Job drawing, mm, ordinate dimensions from the low corner. One solid piece. A direction names the side the tool comes from. Round coordinates to 2 decimals unless told otherwise and drop trailing zeros. Loops run counter-clockwise (first coordinate to the right, second up) from the corner with the lowest first, then second, coordinate; pieces in that order, holes last.
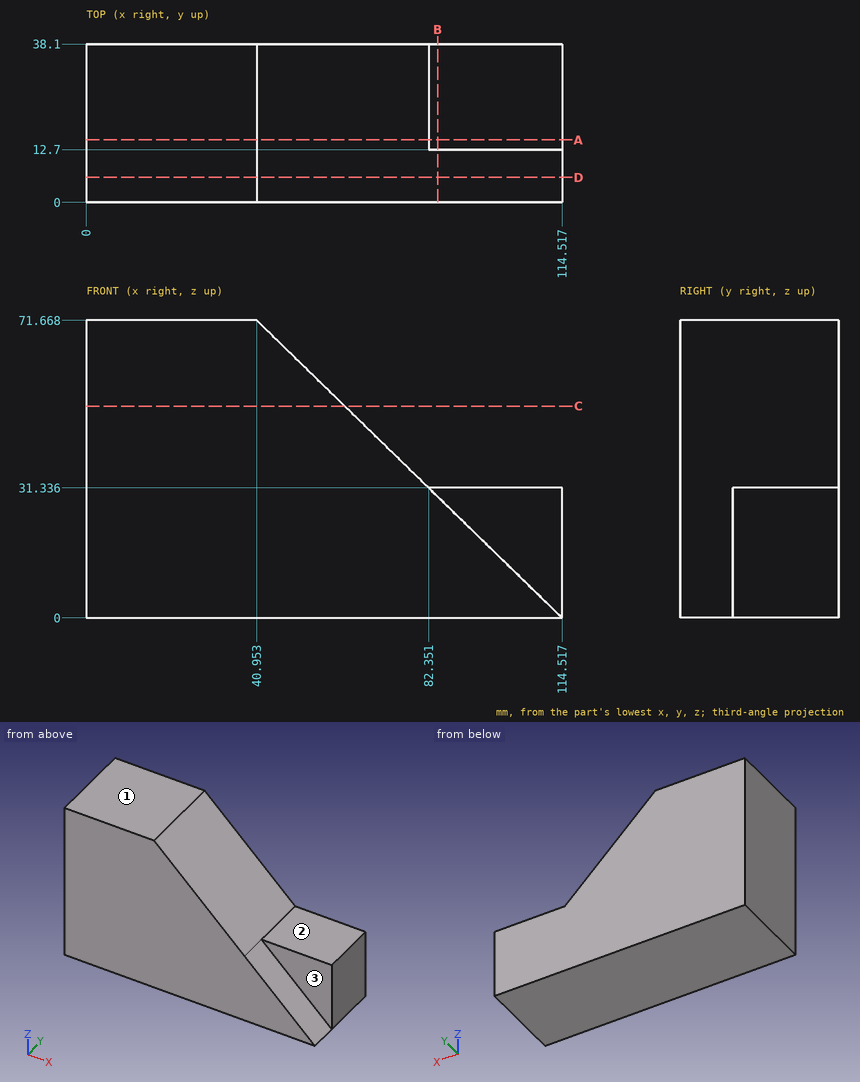
Item 1: Cut at B-B, the plane x = 84.5. Give the cut face in (y, z).
Answers follow:
outline: (0, 0) - (38.1, 0) - (38.1, 31.34) - (12.7, 31.34) - (12.7, 29.24) - (0, 29.24) - close
Item 2: Cut at C-C, the plane z = 51. Give the cut face in (x, y), plus the area to 3 significant figures.
Answers follow:
outline: (0, 0) - (62.17, 0) - (62.17, 38.1) - (0, 38.1) - close
area: 2,370 mm2
Item 3: 3-axis set-ups, long thin cutter, end or side, ignore diameter. For the marked faces 1, 2 and 3: which of +Z, -Z, +X, -X, +Y, -Y reach the whole face in a straight line?
Answers follow:
face 1: +Z, +X, -X, +Y, -Y
face 2: +Z, +X, +Y, -Y
face 3: +Z, +X, -Y
Item 4: Cut at A-A, the plane y = 15. Give the cut face in (x, z), plus the area to 4 significant figures.
Answers follow:
outline: (0, 0) - (114.52, 0) - (114.52, 31.34) - (82.35, 31.34) - (40.95, 71.67) - (0, 71.67) - close
area: 6,075 mm2
Item 5: Probe line 1 (Z direction, x = 104, y = 21); line 2 (Z direction, x = 46, y = 11); line 3 (X direction, y = 24, z = 66). List the from-to ranges inside material, lowest first.
Answers follow:
line 1: z = 0 to 31.34
line 2: z = 0 to 66.75
line 3: x = 0 to 46.77
Item 6: Cut at D-D, the plane y = 6. Give the cut face in (x, z), plus the area to 3 significant figures.
Answers follow:
outline: (0, 0) - (114.52, 0) - (40.95, 71.67) - (0, 71.67) - close
area: 5,570 mm2
Item 7: Flat gauge pins, fed straight in: P1, Ø5, axis at x = 84.5, y = 32.5, coming from the +Z side; P2, Ø7.5, axis at x = 99.5, y = 24.5, coming from the +Z side. Where does each tip first touch, or does it go through?
Answers follow:
P1: stops at z = 31.68
P2: stops at z = 31.34
